Could you check a few things on this drawing? It's one solid part, dimensions in mm from its lowest x, y, z. Give positions to 0.01 mm unless a question says otherwise; leave off trailing zeros. Loops run counter-clockwise (first coordinate to the right, second up) from the corner with the lowest first, then second, coordinate; pieces in that order, holes last. Notation, with made-up numbers: (19, 82) - (29, 82) arc R22 ccw to (29, 105) - close; hole circle Ø8 at (19.5, 1). An arc over 180 degrees is marked (long way). Write each question's results on one line, items separated by ' | '. Start each with the question number.
(1) Suppose I cut it at A-A (y = 17). Count the separate pieces of the cut face and the enclosed holes in it.
(2) Suppose I cut it at B-B (x = 23). Please give me the cut outline in (y, z) (1 decimal).
(3) I need wall thicknesses on line 1 (X direction, y = 20.5, z = 0.5); line 2 (Y direction, x = 15.5, z = 0.1); line 3 (Y direction, x = 42.5, z = 0.9). Which ranges of each line are inside material? Lowest first, please.
(4) Suppose I cut it at D-D (x = 35.5). Please give me the cut outline in (y, z) (1 decimal).
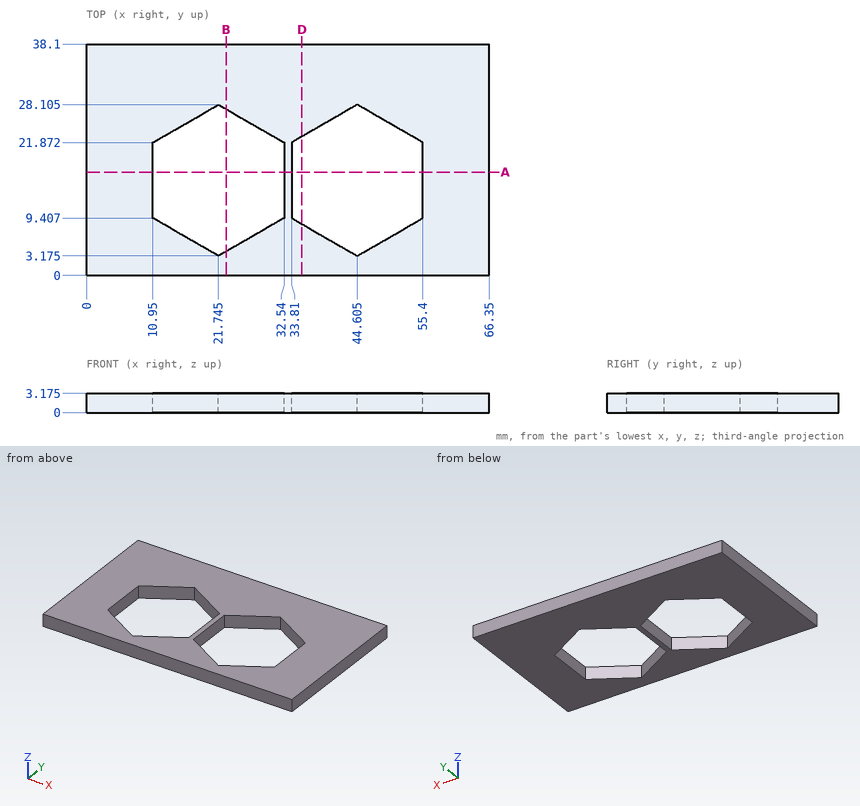
Output values:
1) separate pieces: 3 | enclosed holes: 0
2) outline: (0, 0) - (3.9, 0) - (3.9, 3.2) - (0, 3.2) - close; (27.4, 0) - (38.1, 0) - (38.1, 3.2) - (27.4, 3.2) - close
3) line 1: 0 to 10.95, 32.54 to 33.81, 55.4 to 66.35 | line 2: 0 to 6.78, 24.5 to 38.1 | line 3: 0 to 4.39, 26.89 to 38.1
4) outline: (0, 0) - (8.4, 0) - (8.4, 3.2) - (0, 3.2) - close; (22.8, 0) - (38.1, 0) - (38.1, 3.2) - (22.8, 3.2) - close
